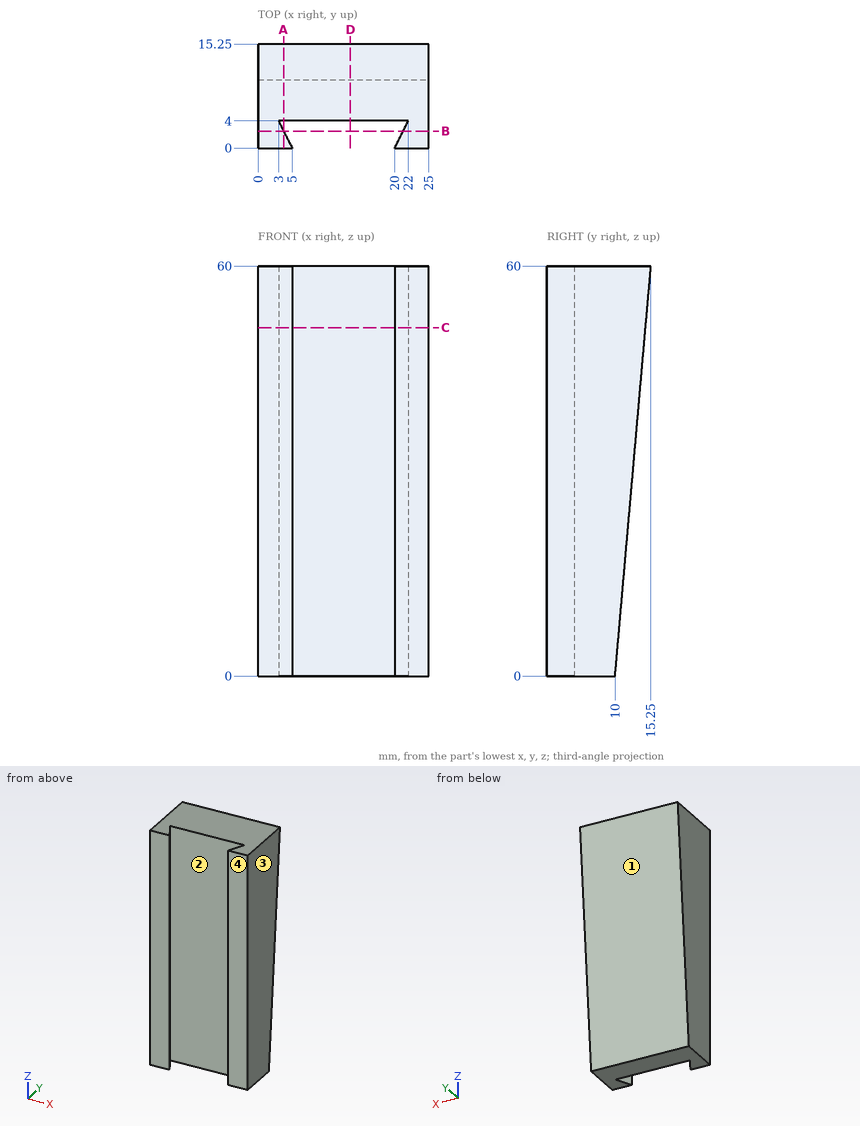
Can you work these out from the drawing? Everything is in mm from the part's minimum corner. Coordinates: 2 decimals unless noted, no trailing zeros. Loops run counter-clockwise (first coordinate to the right, second up) from the corner with the lowest first, then second, coordinate; pieces in that order, holes last.
1. If we mould it in two halves opening along Y, with no side actions, what happens to the marked faces 1, 2, 3 and 4? For each: pulls with the +Y half, pulls with the -Y half, needs draft (parallel to the pull), parting line crosses it, or undercut.
2. Imagine slicing it at A-A, the plane x = 3.75. Please give me the cut outline in (y, z), and give its area (4 significant figures).
3. I need wall thicknesses on L1, parallel to X at y = 1, z = 16.5; L2, parallel to Y at x = 21, z = 49.5; L3, parallel to Y at x = 15.75, z = 15.5. Which ranges of each line are inside material? Lowest first, please.
4. Imagine slicing it at B-B, the plane y = 2.5. Please give me the cut outline in (x, z).
5. Imagine slicing it at D-D, the plane x = 13.5. Please give me the cut outline in (y, z).
6. Imagine slicing it at C-C, the plane z = 51. Please give me the cut outline in (x, y), and give its area (3 significant figures).
7. For P1, Ø9.5, axis at x = 14.5, z = 18.5, coming from the -Y side; P2, Ø10, axis at x = 20, z = 51, coming from the +Y side; P3, Ø5, axis at x = 4.5, z = 41, coming from the +Y side, each with a flat end and sliding along its axis, tell me the tip position at first contact or that it passes through.
Taken from the geometry:
1. face 1: pulls with the +Y half
1. face 2: undercut
1. face 3: needs draft
1. face 4: pulls with the -Y half
2. outline: (0, 0) - (2.5, 0) - (2.5, 60) - (0, 60) - close; (4, 0) - (10, 0) - (15.25, 60) - (4, 60) - close
2. area: 667.5 mm2
3. L1: x = 0 to 4.5, 20.5 to 25
3. L2: y = 0 to 2, 4 to 14.33
3. L3: y = 4 to 11.36
4. outline: (0, 0) - (3.75, 0) - (3.75, 60) - (0, 60) - close; (21.25, 0) - (25, 0) - (25, 60) - (21.25, 60) - close
5. outline: (4, 0) - (10, 0) - (15.25, 60) - (4, 60) - close
6. outline: (0, 0) - (5, 0) - (3, 4) - (22, 4) - (20, 0) - (25, 0) - (25, 14.46) - (0, 14.46) - close
6. area: 294 mm2
7. P1: stops at y = 4
7. P2: stops at y = 14.9
7. P3: stops at y = 13.81
